The model under review builds one solid part; all positions refer to its coordinate system, in mm. Coordinates: 2 decimals unless noted, no trailing zeros. Loops run counter-clockwise (first coordinate to the right, second up) from the corner with the lowest first, then second, coordinate; pieces in that order, holes last. Notation, with made-up numbers: M 1.5,-15 L 44.5,-15 A20 ccw 44.5,24 Z; hole C 78,53 d11. An arc over 180 degrees is marked long. Use one line per item in the form item = value.
```python
from build123d import *

# Parameters (mm, degrees)
SKETCH1_W               = 70
SKETCH1_H               = 35
BOSS_EXTRUDE1_DEPTH     = 2
SKETCH2_R               = 2.5
SKETCH2_R_2             = 1.75
CUT_EXTRUDE1_DEPTH      = 1
CUT_EXTRUDE1_DEPTH_BACK = 3
FILLET1_R               = 1


with BuildPart() as part:
    # Sketch1 → Boss-Extrude1 (new body)
    with BuildSketch(Plane(origin=(0, 0, 0), x_dir=(1, 0, 0), z_dir=(0, 1, 0))):
        with Locations((35, 17.5)):
            Rectangle(SKETCH1_W, SKETCH1_H)
    extrude(amount=BOSS_EXTRUDE1_DEPTH)

    # Sketch2 → Cut-Extrude1 (cut, two sides)
    with BuildSketch(Plane(origin=(0, 2, 0), x_dir=(1, 0, 0), z_dir=(0, 1, 0))) as cut_extrude1_sk:
        with Locations((5, 30)):
            Circle(SKETCH2_R)
        with Locations((5, 5)):
            Circle(SKETCH2_R)
        with Locations((4.25, 17.5)):
            Circle(SKETCH2_R_2)
        with Locations((65.75, 17.5)):
            Circle(SKETCH2_R_2)
        with Locations((65, 5)):
            Circle(SKETCH2_R)
        with Locations((65, 30)):
            Circle(SKETCH2_R)
    extrude(amount=CUT_EXTRUDE1_DEPTH, mode=Mode.SUBTRACT)
    extrude(cut_extrude1_sk.sketch, amount=-CUT_EXTRUDE1_DEPTH_BACK, mode=Mode.SUBTRACT)

    # Fillet1
    fillet1_edges = [part.edges().sort_by_distance(p)[0] for p in [
        (0, 1, -35),
        (70, 1, -35),
        (70, 1, 0),
        (0, 1, 0),
    ]]
    fillet(fillet1_edges, radius=FILLET1_R)


solid = part.part
```
1. Add section A-A (z = -17.5). State the section outline as (x, y) points.
Response values:
outline = M 0,0 L 2.5,0 L 2.5,2 L 0,2 Z; M 6,0 L 64,0 L 64,2 L 6,2 Z; M 67.5,0 L 70,0 L 70,2 L 67.5,2 Z
2. Wall thickness on line 1 along X through (y, z) = (1.15, -17.5); line 2 along X through (y, z) = (1.2, -30); line 3 along Z through (x, y) = (5, 1.35): over which ranges is each line inside the solid? List them lowest first. Write a range as from..to.
Response values:
line_1 = 0..2.5, 6..64, 67.5..70
line_2 = 0..2.5, 7.5..62.5, 67.5..70
line_3 = -35..-32.5, -27.5..-19.08, -15.92..-7.5, -2.5..0
3. The part is to be moulded in two halves that separate along X. For faces 1 (the face through (35, 1, -35)), 2 (the face through (67.419, 1.014, -18.026)), 3 (the face through (0, 1, -17)), say which applies: pulls with the +X half, pulls with the -X half, needs draft (parallel to the pull), parting line crosses it, or undercut.
Response values:
face_1 = needs draft
face_2 = undercut
face_3 = pulls with the -X half
4. Add section C-C (x = 65.75). State the section outline as (y, z) points.
Response values:
outline = M 0,-35 L 2,-35 L 2,-32.38 L 0,-32.38 Z; M 0,-27.62 L 2,-27.62 L 2,-19.25 L 0,-19.25 Z; M 0,-15.75 L 2,-15.75 L 2,-7.38 L 0,-7.38 Z; M 0,-2.62 L 2,-2.62 L 2,0 L 0,0 Z
5. Add section B-B (y = 1.65). State the section outline as (x, z) points.
Response values:
outline = M 0,-34 A1 ccw 1,-35 L 69,-35 A1 ccw 70,-34 L 70,-1 A1 ccw 69,0 L 1,0 A1 ccw 0,-1 Z; hole C 5,-30 d5; hole C 4.25,-17.5 d3.5; hole C 5,-5 d5; hole C 65,-30 d5; hole C 65,-5 d5; hole C 65.75,-17.5 d3.5
6. Add section D-D (z = -5). State the section outline as (x, y) points, then the cut area to 3 significant figures.
Response values:
outline = M 0,0 L 2.5,0 L 2.5,2 L 0,2 Z; M 7.5,0 L 62.5,0 L 62.5,2 L 7.5,2 Z; M 67.5,0 L 70,0 L 70,2 L 67.5,2 Z
area = 120 mm^2
